Verification items for the finished model (mm, model axes). A direction names the side the tool comes from. Coordinates: 2 decimals unless noted, no trailing zeros. Order: outer loops, then holes, each group sorted by start corner. A loop starts at its lowest first (then second) coordinate and runs counter-clockwise, first axis right, second up. Notation, with made-up numbers: M -36.75,40.25 L -28.75,40.25 A10 ccw -28.75,54.25 Z; hole C 36,86.5 d10. An arc over 180 degrees is marked long. Use one line per item in the form item = value. Start each with the question number.
```python
from build123d import *

# Parameters (mm, degrees)
F1_DEPTH = 10
F2_R     = 1.5875
F4_DEPTH = 9


with BuildPart() as f1:
    # F0 (on Top) → F1 (new body)
    with BuildSketch(Plane.XY):
        with BuildLine():
            ThreePointArc((42.0751, 54.7751), (38.355356, 63.755356), (29.3751, 67.4751))
            Line((29.3751, 67.4751), (-29.3751, 67.4751))
            ThreePointArc((-29.3751, 67.4751), (-38.355356, 63.755356), (-42.0751, 54.7751))
            Line((-42.0751, 54.7751), (-42.0751, -54.7751))
            ThreePointArc((-42.0751, -54.7751), (-38.355356, -63.755356), (-29.3751, -67.4751))
            Line((-29.3751, -67.4751), (29.3751, -67.4751))
            ThreePointArc((29.3751, -67.4751), (38.355356, -63.755356), (42.0751, -54.7751))
            Line((42.0751, -54.7751), (42.0751, 54.7751))
        make_face()
    extrude(amount=F1_DEPTH)

    # F2
    f2_edges = [f1.edges().sort_by_distance(p)[0] for p in [
        (42.0751, 0, 10),
        (38.355356, -63.755356, 10),
        (0, -67.4751, 10),
        (-38.355356, -63.755356, 10),
        (-42.0751, 0, 10),
        (-38.355356, 63.755356, 10),
        (0, 67.4751, 10),
        (38.355356, 63.755356, 10),
    ]]
    fillet(f2_edges, radius=F2_R)

    # F3 (on Top) → F4 (cut)
    with BuildSketch(Plane.XY):
        with BuildLine():
            Line((-28.575, -66.675), (28.575, -66.675))
            ThreePointArc((28.575, -66.675), (37.555256, -62.955256), (41.275, -53.975))
            Line((41.275, -53.975), (41.275, 53.975))
            ThreePointArc((41.275, 53.975), (37.555256, 62.955256), (28.575, 66.675))
            Line((28.575, 66.675), (-28.575, 66.675))
            ThreePointArc((-28.575, 66.675), (-37.555256, 62.955256), (-41.275, 53.975))
            Line((-41.275, 53.975), (-41.275, -53.975))
            ThreePointArc((-41.275, -53.975), (-37.555256, -62.955256), (-28.575, -66.675))
        make_face()
    extrude(amount=F4_DEPTH, mode=Mode.SUBTRACT)


solid = f1.part
```
1. Cross-section at C-C on x = -18. Enter the section's corners in (y, z) (1 decimal).
2. Depth check by flat-ended pin: P1, Ø6, axis at x = -27.5, y = -48, coming from the -Z side. Enter the tip coordinate at first touch or a pass-through.
3. Tool access check on faces 1 (the flat face through (41.275, -1, 4)), 2 (the cylindrical face through (38.45, 63.66, 4.15)). Record the directions out of +Z, -Z, +X, -X, +Y, -Y that give a thin tool (end or side, any length) a straight path to the whole face; none if there is none.
4. Cross-section at A-A on y = 16. Enter the section's corners in (x, z) (1 decimal).
5. Material ranges on line 1 along Y through (x, z) = (-4.5, 6.5) (3 decimals); line 2 along X through (y, z) = (-17, 8) (3 decimals); line 3 along Z through (x, y) = (-38, -26), recorded low to high.
6. Cross-section at B-B on z = 1.75. Enter the section's corners in (x, y) (3 decimals).
7. Release check for a two-part mould opening along Y. For faces 3 (the flat face through (-41.275, 1, 4)), 4 (the flat face through (0, 67.475, 4)), 5 (the flat face through (-42.075, 1, 4)), 6 (the cylindrical face through (38.26, -63.85, 4.15)) record: pulls with the +Y half, pulls with the -Y half, needs draft (parallel to the pull), parting line crosses it, or undercut.
Final values:
q1.outline = M -67.5,0 L -66.7,0 L -66.7,9 L 66.7,9 L 66.7,0 L 67.5,0 L 67.5,8.4 A1.6 ccw 65.9,10 L -65.9,10 A1.6 ccw -67.5,8.4 Z
q2.P1 = 9
q3.face_1 = -Z
q3.face_2 = +Z, -Z, +X, +Y
q4.outline = M -42.1,0 L -41.3,0 L -41.3,9 L 41.3,9 L 41.3,0 L 42.1,0 L 42.1,8.4 A1.6 ccw 40.5,10 L -40.5,10 A1.6 ccw -42.1,8.4 Z
q5.line_1 = -67.475 to -66.675, 66.675 to 67.475
q5.line_2 = -42.075 to -41.275, 41.275 to 42.075
q5.line_3 = 9 to 10
q6.outline = M -42.075,-54.775 A12.7 ccw -29.375,-67.475 L 29.375,-67.475 A12.7 ccw 42.075,-54.775 L 42.075,54.775 A12.7 ccw 29.375,67.475 L -29.375,67.475 A12.7 ccw -42.075,54.775 Z; hole M -41.275,-53.975 A12.7 ccw -28.575,-66.675 L 28.575,-66.675 A12.7 ccw 41.275,-53.975 L 41.275,53.975 A12.7 ccw 28.575,66.675 L -28.575,66.675 A12.7 ccw -41.275,53.975 Z
q7.face_3 = undercut
q7.face_4 = pulls with the +Y half
q7.face_5 = needs draft
q7.face_6 = pulls with the -Y half
